Can you work these out from the model? Positions are in its coordinate system, mm. A direction names the side the tool comes from. Round coordinates to 2 decimals unless told otherwise and drop trailing zeros. Loops run counter-clockwise (first coordinate to the right, second up) from the corner with the lowest first, then second, coordinate; pieces in that order, holes last. Notation, with made-up numbers: (28.5, 60.25) - (77.5, 60.25) arc R33 ccw to (77.5, 99.25) - close; hole circle Ø4 at (-16, -25). An arc over 180 degrees is marked (long way). Answer as CSV lines item,"result".
```python
from build123d import *

# Parameters (mm, degrees)
BOSS_EXTRUDE2_DEPTH = 287.5
SHELL1_START        = -267.5
SHELL1_DEPTH        = 535
SKETCH4_R           = 15
BOSS_EXTRUDE3_DEPTH = 55
BOSS_EXTRUDE4_DEPTH = 287.5
BOSS_EXTRUDE5_START = 75
SKETCH6_R           = 30
BOSS_EXTRUDE5_DEPTH = 20
BOSS_EXTRUDE6_DEPTH = 48
CUT_EXTRUDE1_DEPTH  = 849.457518617
LPATTERN1_COUNT     = 4
LPATTERN1_PITCH     = 107


# Read off the part's stored shape, not the designer's step: Shell1
with BuildPart() as part:
    # Sketch1 → Boss-Extrude2 (new, symmetric)
    with BuildSketch(Plane(origin=(0, 0, 0), x_dir=(0, 0, -1), z_dir=(1, 0, 0))):
        with BuildLine():
            Line((-17.131272745, -20.34711833), (18.677931789, 22.184112876))
            Line((18.677931789, 22.184112876), (-45.510379426, 47.499339584))
            Line((-45.510379426, 47.499339584), (-11.452124758, 96.896052925))
            Line((-11.452124758, 96.896052925), (77.065235948, 113.164945136))
            Line((77.065235948, 113.164945136), (286.140990264, 434.746925642))
            Line((286.140990264, 434.746925642), (400.489865708, 393.127338659))
            ThreePointArc((400.489865708, 393.127338659), (527.907623498, 152.23232826), (317, -20.34711833))
            Line((317, -20.34711833), (-17.131272745, -20.34711833))
        make_face()
    extrude(amount=BOSS_EXTRUDE2_DEPTH, both=True)

    # Shell1 outline → Shell1 (cut)
    with BuildSketch(Plane.YZ.offset(SHELL1_START)):
        with BuildLine():
            Line((-0.34711833, 0.292256559), (-0.347118332, -316.999753995))
            ThreePointArc((-0.347118332, -316.999753995), (155.954494492, -508.255406969), (374.506719993, -393.173507026))
            Line((374.506719993, -393.173507026), (417.536054052, -274.951383325))
            Line((417.536054052, -274.951383325), (113.164945136, -77.065235948))
            Line((113.164945136, -77.065235948), (96.896052925, 11.452124758))
            Line((96.896052925, 11.452124758), (47.499339584, 45.510379426))
            Line((47.499339584, 45.510379426), (22.184112876, -18.677931789))
            Line((22.184112876, -18.677931789), (-0.34711833, 0.292256559))
        make_face()
    extrude(amount=SHELL1_DEPTH, mode=Mode.SUBTRACT)

    # Sketch4 → Boss-Extrude3 (add, symmetric)
    with BuildSketch(Plane(origin=(0, 0, 0), x_dir=(0, 0, -1), z_dir=(1, 0, 0))):
        with BuildLine():
            Line((473.490355169, 471.5), (422.135414248, 382.550633104))
            ThreePointArc((422.135414248, 382.550633104), (443.346279027, 368.983010842), (462.826942921, 353.030428204))
            Line((462.826942921, 353.030428204), (516.791625358, 446.5))
            ThreePointArc((516.791625358, 446.5), (507.640990264, 480.650635095), (473.490355169, 471.5))
        make_face()
        with Locations((495.140990264, 459)):
            Circle(SKETCH4_R, mode=Mode.SUBTRACT)
    extrude(amount=BOSS_EXTRUDE3_DEPTH, both=True)

    # Sketch5 → Boss-Extrude4 (add, symmetric)
    with BuildSketch(Plane(origin=(0, 0, 0), x_dir=(0, 0, -1), z_dir=(1, 0, 0))):
        with BuildLine():
            Line((286.140990264, 434.746925642), (384.921412729, 398.793792137))
            ThreePointArc((384.921412729, 398.793792137), (341.171815777, 432.267819258), (286.140990264, 434.746925642))
        make_face()
    extrude(amount=BOSS_EXTRUDE4_DEPTH, both=True)

    # Sketch6 → Boss-Extrude5 (add)
    with BuildSketch(Plane(origin=(0, 0, 0), x_dir=(0, 0, -1), z_dir=(1, 0, 0)).offset(BOSS_EXTRUDE5_START)):
        with BuildLine():
            ThreePointArc((364.02781167, 579.815744274), (307.663748085, 590.61449937), (278.276573516, 541.320333932))
            Line((278.276573516, 541.320333932), (286.140990264, 434.746925642))
            ThreePointArc((286.140990264, 434.746925642), (341.171815777, 432.267819258), (384.921412729, 398.793792137))
            Line((384.921412729, 398.793792137), (400.489865708, 393.127338659))
            ThreePointArc((400.489865708, 393.127338659), (487.746891868, 325.745206641), (530.177667873, 223.99173212))
            ThreePointArc((530.177667873, 223.99173212), (477.038065131, 415.881856126), (364.02781167, 579.815744274))
        make_face()
        with Locations((328.140990264, 545)):
            Circle(SKETCH6_R, mode=Mode.SUBTRACT)
    boss_extrude5 = extrude(amount=-BOSS_EXTRUDE5_DEPTH)

    # Mirror1: Boss-Extrude5 across plane
    add(boss_extrude5.mirror(Plane(origin=(0, 0, 0), x_dir=(0, 0, 1), z_dir=(1, 0, 0))))

    # Sketch9 → Boss-Extrude6 (add)
    with BuildSketch(Plane(origin=(-184.5, 0, 0), x_dir=(0, 0, -1), z_dir=(1, 0, 0))):
        Polygon((-2.207998194, -40.938965281), (-7.30496659, -40.938965281), (-7.744921849, -38.400642166), (-78.864458205, -49.626128726), (-147.468055977, -50.72115136), (-147.941109389, -48.777901384), (-84.440877624, -20.13490752), (-26.871687982, -11.048203673), (-26.183722798, -13.874286929), (-20.257094768, -12.938829716), (-10.765705608, -4.578537278), (-4.89400709, -5.81269955), (-17.131272745, -20.34711833), (62.868727255, -20.34711833), (63.601430642, -34.327931817), (5.327818547, -43.557565254), align=None)
    boss_extrude6 = extrude(amount=BOSS_EXTRUDE6_DEPTH)

    # Sketch10 → Cut-Extrude1 (cut, symmetric)
    with BuildSketch(Plane(origin=(0, 0, 0), x_dir=(1, 0, 0), z_dir=(0, 1, 0))):
        Polygon((-184.5, -123.07463289), (-162.5, -147.941109389), (-184.5, -147.941109389), align=None)
        Polygon((-158.5, -147.941109389), (-136.5, -123.07463289), (-136.5, -147.941109389), align=None)
    cut_extrude1 = extrude(amount=CUT_EXTRUDE1_DEPTH, both=True, mode=Mode.SUBTRACT)

    # LPattern1: Boss-Extrude6, Cut-Extrude1 ×4
    with Locations(*[(i * LPATTERN1_PITCH, 0, 0) for i in range(1, LPATTERN1_COUNT)]):
        add(boss_extrude6)
        add(cut_extrude1, mode=Mode.SUBTRACT)


solid = part.part
```
Q1. Imagine slicing it at D-D (y = 11). Write out the boundary of the cut face in (x, z), then the cut area to 3 significant figures.
Checks:
outline,"(-287.5, -428.83) - (287.5, -428.83) - (287.5, -9.26) - (267.5, -9.26) - (267.5, -382.57) - (-267.5, -382.57) - (-267.5, -9.26) - (-287.5, -9.26) - close"
area,"41,500 mm²"
Q2. Imagine slicing it at B-B (x = -225.5). Write out the boundary of the cut face in (y, z).
Checks:
outline,"(-20.35, -317) arc R215.17 ccw to (393.13, -400.49) - (398.79, -384.92) arc R92 ccw to (434.75, -286.14) - (417.54, -274.95) - (374.51, -393.17) arc R195.17 cw to (-0.35, -317) - (-0.35, 0.29) - (-20.35, 17.13) - close"
Q3. On a 3-axis mill with a long thin cutter (end or side, diameter ignored), from which of +Z, -Z, +X, -X, +Y, -Y can I reach the whole of each face in a straight line? I mean faces 1 (the cylindrical face through (4.025, 156.29, -528.686)), 2 (the cylindrical face through (-3.745, 152.293, -507.475)), 3 (the flat face through (277.64, 71.85, 28.72)), 4 (the flat face through (55, 490, -368)). Say none if no direction works.
Checks:
face 1,"-Z"
face 2,"+Z"
face 3,"+Z, +X, -X, +Y"
face 4,"+Y"
Q4. Imagine slicing it at C-C (y = 243). Write out the boundary of the cut face in (x, z).
Checks:
outline,"(-287.5, -526.7) - (-75, -526.7) - (-75, -527.9) - (-55, -527.9) - (-55, -526.7) - (55, -526.7) - (55, -527.9) - (75, -527.9) - (75, -526.7) - (287.5, -526.7) - (287.5, -161.48) - (267.5, -161.48) - (267.5, -506.12) - (-267.5, -506.12) - (-267.5, -161.48) - (-287.5, -161.48) - close"
Q5. We'd pull the mould along Y, two halves only. Please class faces 5 (the flat face through (-3.75, 395.72, -334.89)), 6 (the flat face through (-55, 490, -368)), 7 (the cylindrical face through (0.8, 432, -341.9)), 8 (the flat face through (160.164, -43.935, 42.807)): pulls with the +Y half, pulls with the -Y half, needs draft (parallel to the pull), parting line crosses it, or undercut.
Checks:
face 5,"undercut"
face 6,"needs draft"
face 7,"pulls with the +Y half"
face 8,"pulls with the -Y half"
Q6. I'm going to push flat-ended pins straight in: pin 1 Ø23 at (y, z) = (-38, 13.5) entering from +X; pin 2 Ø23 at (y, z) = (-22.5, 49) entering from -X; pin 3 Ø1.5 at (x, y) = (148.5, 127.5) entering from +Z. Where does each tip first touch, or does it pass through?
Checks:
pin 1,"x = 184.5"
pin 2,"x = -184.5"
pin 3,"z = -499.91"
Q7. If I drill on line 1 along X through (y, z) = (215.5, -193.5); line 2 along Y through (x, z) = (14, -289); line 3 along Y through (x, z) = (-238, -256), over which ranges is the centre line in solid material (lowest first)? Write a range as [from, to].
Checks:
line 1,"[-287.5, -267.5], [267.5, 287.5]"
line 2,"[-20.35, -0.35], [412.42, 435.46]"
line 3,"[-20.35, -0.35]"
Q8. Imagine slicing it at A-A (y = 459). Write out the boundary of the cut face in (x, z).
Checks:
outline,"(-75, -454.74) - (-55, -454.74) - (-55, -284.35) - (-75, -284.35) - close; (-55, -520.14) - (55, -520.14) - (55, -510.14) - (-55, -510.14) - close; (-55, -480.14) - (55, -480.14) - (55, -466.27) - (-55, -466.27) - close; (55, -454.74) - (75, -454.74) - (75, -284.35) - (55, -284.35) - close"
